Check sheet for the modelled part. Datum: model origin and axes. Units: mm. Give positions to 0.01 mm unless a question says otherwise; leave off trailing zeros. Write each loop counter-clockwise with the first axis right and the second up, starting at its lowest first coordinate (ties: lowest second). Pieces come first, ordered by that corner, then holes. Notation, with made-up numbers: (8, -27) -> (39, -27) arc R20 cw to (39, -20) -> close; hole circle Ø3 at (33, 34.5). An arc over 180 degrees is marked (long way). Use a Markdown table: item, result. Add a question column.
1. Cross-section at B-B (y = 15.95). Enter the section's corners in (x, z).
2. Scan lines: probe 1 along Z at (x, y) = (7.5, 15.35); probe 2 along Y at (x, z) = (28, 37.2); probe 3 along Z at (x, y) = (10.5, 14.3). Record each from-to range of solid material in increasing order. Write a range as [from, to].
3. Cross-section at A-A (x = 21). Enter the section's corners in (y, z) (3 decimals), then the cut area to 3 significant figures.
4. Cross-section at C-C (x = 38.5). Enter the section's corners in (y, z) (3 decimals), then the cut area to 3 significant figures.
5. Gauge pin test, flat ends, axial feed: P1, Ø0.7, axis at x = 14.5, z = 36, coming from the -Y side; P2, Ø1, axis at x = 10.5, y = 14, coming from the +Z side; P3, Ø0.5, axis at x = 15.5, z = 35.5, coming from the +Y side. Record the tip position at first contact, or that the pin passes through.
6. Release check for a two-part mould opening along Z. For faces 1 (the cylindrical face through (21.91, 15.43, 36.08)), 2 (the flat face through (0, 16.5, 37.3)), 3 (the cylindrical face through (21.914, 15.622, 35.474)) record: released by +Z, released by -Z, zero draft, split by the parting line, or undercut.
from build123d import *

# Parameters (mm, degrees)
SKETCH1_R               = 1.905
SKETCH1_R_2             = 1.27
BOSS_EXTRUDE1_DEPTH     = 44.45
CUT_EXTRUDE6_DEPTH      = 8.382
CUT_EXTRUDE6_DEPTH_BACK = 6.858


with BuildPart() as part:
    # Sketch1 → Boss-Extrude1 (new body)
    with BuildSketch(Plane(origin=(0, 0, 0), x_dir=(0, 0, -1), z_dir=(1, 0, 0))):
        with Locations((-37.290755903, 15.049483632)):
            Circle(SKETCH1_R)
        with Locations((-37.290755903, 15.049483632)):
            Circle(SKETCH1_R_2, mode=Mode.SUBTRACT)
    extrude(amount=BOSS_EXTRUDE1_DEPTH)

    # Sketch10 → Cut-Extrude6 (cut, two sides: drawn at the far end of the back side and taken through both)
    with BuildSketch(Plane.XY.offset(39.195755903).offset(-CUT_EXTRUDE6_DEPTH_BACK)):
        Polygon((0, 15.049483632), (0, 15.252683632), (33.032460862, 15.252683632), (33.032460862, 15.007269714), (33.032460862, 14.846283632), (0, 14.846283632), align=None)
    extrude(amount=CUT_EXTRUDE6_DEPTH + CUT_EXTRUDE6_DEPTH_BACK, mode=Mode.SUBTRACT)


solid = part.part
Worked answers:
| question | item | result |
|---|---|---|
| 1 | outline | (0, 35.61) -> (44.45, 35.61) -> (44.45, 36.4) -> (0, 36.4) -> close; (0, 38.19) -> (44.45, 38.19) -> (44.45, 38.97) -> (0, 38.97) -> close |
| 2 | probe 1 | z = [35.41, 36.06], [38.52, 39.17] |
| 2 | probe 2 | y = [13.15, 13.78], [16.32, 16.95] |
| 2 | probe 3 | z = [35.54, 36.27], [38.32, 39.04] |
| 3 | outline | (14.846, 35.397) -> (14.846, 36.037) arc R1.27 cw to (14.846, 38.544) -> (14.846, 39.185) arc R1.905 ccw to start; (15.253, 35.397) arc R1.905 ccw to (15.253, 39.185) -> (15.253, 38.544) arc R1.27 cw to (15.253, 36.037) -> close |
| 3 | area | 5.82 mm² |
| 4 | outline | circle Ø3.81 at (15.049, 37.291); hole circle Ø2.54 at (15.049, 37.291) |
| 4 | area | 6.33 mm² |
| 5 | P1 | stops at y = 13.39 |
| 5 | P2 | stops at z = 39.11 |
| 5 | P3 | stops at y = 16.17 |
| 6 | face 1 | undercut |
| 6 | face 2 | zero draft |
| 6 | face 3 | split by the parting line |
